Check sheet for the modelled part. Datum: model origin and axes. Units: mm. Give positions to 0.01 mm unless a question says otherwise; leave off trailing zeros. Order: outer loops, then holes, each group sorted by start corner. A loop starts at its lowest first (then second) coordinate and runs counter-clockwise, first axis right, second up.
```python
from build123d import *

# Parameters (mm, degrees)
SKETCH1_W           = 1219.2
SKETCH1_H           = 1771.65
BOSS_EXTRUDE1_DEPTH = 19.05
SKETCH2_W           = 869.95
SKETCH2_H           = 534.9875
CUT_EXTRUDE1_DEPTH  = 20.05
SKETCH3_W           = 80.9625
SKETCH3_H           = 685.8
CUT_EXTRUDE2_DEPTH  = 20.05
SKETCH4_W           = 676.20134
SKETCH4_H           = 863.85146
CUT_EXTRUDE3_DEPTH  = 20.05
CUT_EXTRUDE4_DEPTH  = 1220.2
CHAMFER1_SIZE       = 2.032


with BuildPart() as part:
    # Sketch1 → Boss-Extrude1 (new body)
    with BuildSketch(Plane(origin=(0, 0, 0), x_dir=(1, 0, 0), z_dir=(0, 1, 0))):
        with Locations((609.6, 885.825)):
            Rectangle(SKETCH1_W, SKETCH1_H)
    extrude(amount=-BOSS_EXTRUDE1_DEPTH)

    # Sketch2 → Cut-Extrude1 (cut, through all)
    with BuildSketch(Plane(origin=(0, 0, 0), x_dir=(1, 0, 0), z_dir=(0, 1, 0))):
        with Locations((697.865, 318.29375)):
            Rectangle(SKETCH2_W, SKETCH2_H)
    extrude(amount=-CUT_EXTRUDE1_DEPTH, mode=Mode.SUBTRACT)

    # Sketch3 → Cut-Extrude2 (cut, through all)
    with BuildSketch(Plane(origin=(0, 0, 0), x_dir=(1, 0, 0), z_dir=(0, 1, 0))):
        with Locations((40.48125, 342.9)):
            Rectangle(SKETCH3_W, SKETCH3_H)
    extrude(amount=-CUT_EXTRUDE2_DEPTH, mode=Mode.SUBTRACT)

    # Sketch4 → Cut-Extrude3 (cut, through all)
    with BuildSketch(Plane(origin=(0, 0, 0), x_dir=(1, 0, 0), z_dir=(0, 1, 0))):
        with Locations((695.28817, 1260.98427)):
            Rectangle(SKETCH4_W, SKETCH4_H)
    extrude(amount=-CUT_EXTRUDE3_DEPTH, mode=Mode.SUBTRACT)

    # Sketch5 → Cut-Extrude4 (cut, through all)
    with BuildSketch(Plane.ZY):
        Polygon((-1436.1414, 0), (-1417.0914, 0), (-1417.0914, -5.969), (-1414.4244, -5.969), (-1414.4244, -9.525), (-1438.8084, -9.525), (-1438.8084, -5.969), (-1436.1414, -5.969), align=None)
    extrude(amount=-CUT_EXTRUDE4_DEPTH, mode=Mode.SUBTRACT)

    # Chamfer1
    chamfer1_edges = [part.edges().sort_by_distance(p)[0] for p in [
        (1132.84, 0, -318.29375),
        (697.865, 0, -585.7875),
        (262.89, 0, -318.29375),
        (697.865, 0, -50.8),
        (650.08125, 0, 0),
        (80.9625, 0, -342.9),
        (40.48125, 0, -685.8),
        (1033.38884, 0, -1123.07497),
        (695.28817, 0, -1692.91),
        (357.1875, 0, -1564.5257),
        (695.28817, 0, -829.05854),
        (609.6, 0, -1771.65),
        (1219.2, 0, -708.5457),
        (357.1875, 0, -1123.07497),
        (1033.38884, 0, -1564.5257),
        (1219.2, 0, -1603.8957),
    ]]
    chamfer(chamfer1_edges, length=CHAMFER1_SIZE)


solid = part.part
```
(1) Material ranges on L1, parallel to Z at x = 987, y = -7.25; L2, parallel to Z at x = 1106.5, y = -7.5; L3, parallel to X at y = -9.5, z = -477, recorded low to high.
Response values:
L1: z = -1771.65 to -1692.91, -829.06 to -585.79, -50.8 to 0
L2: z = -1771.65 to -1438.81, -1414.42 to -585.79, -50.8 to 0
L3: x = 80.96 to 262.89, 1132.84 to 1219.2
(2) Gauge pin test, flat end, axial feed: pin 1 Ø1.5 at (y, z) = (-10, -668) entering from -X. Record the tip position at first contact, or that the pin passes through.
Response values:
pin 1: stops at x = 80.96
(3) Cross-section at C-C on x = 473. Enter the section's corners in (y, z).
Response values:
outline: (-19.05, -1771.65) - (-2.03, -1771.65) - (0, -1769.62) - (0, -1694.94) - (-2.03, -1692.91) - (-19.05, -1692.91) - close; (-19.05, -829.06) - (-2.03, -829.06) - (0, -827.03) - (0, -587.82) - (-2.03, -585.79) - (-19.05, -585.79) - close; (-19.05, -50.8) - (-2.03, -50.8) - (0, -48.77) - (0, -2.03) - (-2.03, 0) - (-19.05, 0) - close
(4) Cross-section at D-D on z = -1366. Enter the section's corners in (x, y).
Response values:
outline: (0, -19.05) - (357.19, -19.05) - (357.19, -2.03) - (355.16, 0) - (0, 0) - close; (1033.39, -19.05) - (1219.2, -19.05) - (1219.2, -2.03) - (1217.17, 0) - (1035.42, 0) - (1033.39, -2.03) - close
(5) Cross-section at B-B on z = -415.5. Enter the section's corners in (x, y), then the cut area to 3 significant figures.
Response values:
outline: (80.96, -19.05) - (262.89, -19.05) - (262.89, -2.03) - (260.86, 0) - (82.99, 0) - (80.96, -2.03) - close; (1132.84, -19.05) - (1219.2, -19.05) - (1219.2, -2.03) - (1217.17, 0) - (1134.87, 0) - (1132.84, -2.03) - close
area: 5,100 mm2
